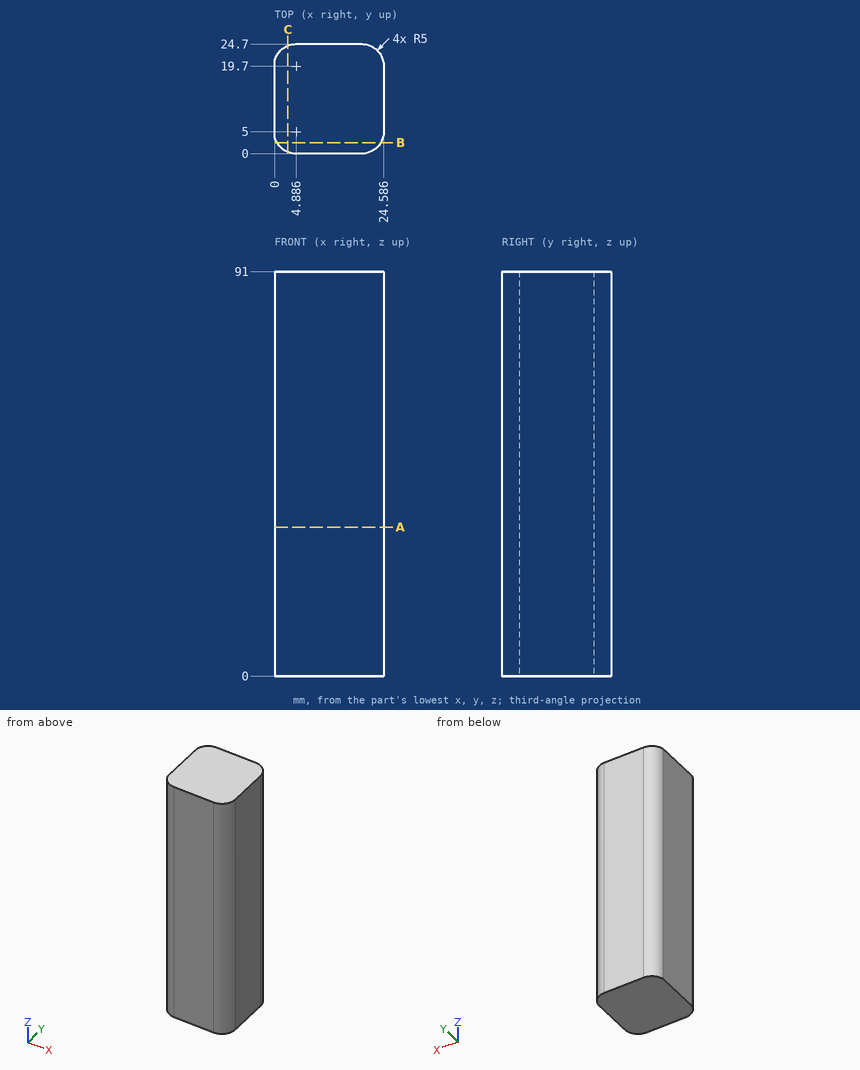
Check sheet for the drawn part. Datum: minimum x, y, z corner. Units: mm. Round coordinates to 2 decimals unless told otherwise and drop trailing zeros. Order: outer loops, then holes, each group sorted by start corner. A loop starts at its lowest first (then second) coordinate and runs counter-clockwise, first axis right, second up. Notation, with made-up numbers: (23.25, 19.5) -> (43.25, 19.5) arc R30 cw to (43.25, 47.5) -> close; hole circle Ø5 at (29, 60.25). An arc over 180 degrees is marked (long way). Return JSON: item names as keys, results as strings. Group by question number.
Q1. Section check A-A, the plane z = 33.5. Record the boundary of the cut face in (x, y).
Q2. Material ranges on probe 1 along X at (y, z) = (4, 83) (1 decimal); probe 2 along X at (y, z) = (21, 58.5) (1 decimal); probe 3 along Y at (x, z) = (20.25, 49) (1 decimal), recorded low to high. Write a range as from..to.
Q3. Section check C-C, the plane x = 3. Record the boundary of the cut face in (y, z), plus the area to 3 significant figures.
Q4. Section check B-B, the plane y = 2.5. Record the boundary of the cut face in (x, z).
Q5. Gauge pin test, flat end, axial feed: pin 1 (1 mm diameter, centred on y = 21.5, z = 69, fed in from -X). Record the tip position at first contact, or that the pin passes through.
Numbers:
{
 "1": {"outline": "(0, 3.94) arc R5 ccw to (4.89, 0) -> (19.59, 0) arc R5 ccw to (24.59, 5) -> (24.59, 19.7) arc R5 ccw to (19.59, 24.7) -> (4.89, 24.7) arc R5 ccw to (0, 20.76) -> close"},
 "2": {"probe 1": "0..24.5", "probe 2": "0.1..24.4", "probe 3": "0..24.7"},
 "3": {"outline": "(0.37, 0) -> (24.33, 0) -> (24.33, 91) -> (0.37, 91) -> close", "area": "2,180 mm^2"},
 "4": {"outline": "(0.56, 0) -> (23.92, 0) -> (23.92, 91) -> (0.56, 91) -> close"},
 "5": {"pin 1": "x = 0.06"}
}
